Read the model definition and answer for the solid it produces. Units are mm, in the model's axes. Coordinates: 2 decimals unless noted, no trailing zeros. Answer as a JSON object with one key per item and string values. Group by question number.
1) Given pin 1 (6 mm diameter, centred on x = 0, y = 196, fed in from -Z), flat-ended and moving along its own axis, determine where the tip first touches the part or whether it passes through.
2) Consider L1, parallel to Y at x = 12, z = 1.55; L2, parallel to X at y = -224, z = 3; L3, parallel to X at y = -216, z = 3. Determine where each line is inside the solid, lowest interval first.
3) Section A-A on z = 4.2 is taken. Count the separate pieces of the cut face and the enclosed holes in it, and give its area (3 significant figures).
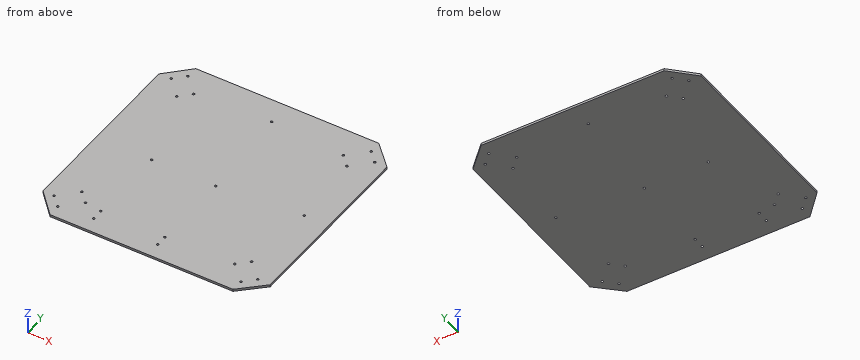
from build123d import *

# Parameters (mm, degrees)
SKETCH2_W           = 500
SKETCH2_H           = 500
BOSS_EXTRUDE1_DEPTH = 5
CUT_EXTRUDE1_DEPTH  = 5
SKETCH4_R           = 2.5
CUT_EXTRUDE4_DEPTH  = 6
SKETCH6_R           = 2.5
CUT_EXTRUDE5_DEPTH  = 6
SKETCH6_3_R         = 2.5
CUT_EXTRUDE6_DEPTH  = 6
SKETCH7_R           = 2.5
CUT_EXTRUDE7_DEPTH  = 6


with BuildPart() as part:
    # Sketch2 → Boss-Extrude1 (new body)
    with BuildSketch(Plane.XY):
        Rectangle(SKETCH2_W, SKETCH2_H)
    extrude(amount=BOSS_EXTRUDE1_DEPTH)

    # Sketch3 → Cut-Extrude1 (cut)
    with BuildSketch(Plane.XY.offset(5)):
        Polygon((-250, 250), (-250, 200.502525317), (-200.502525317, 250), align=None)
        Polygon((250, 250), (200.502525317, 250), (250, 200.502525317), align=None)
        Polygon((250, -202.085866883), (198.968285864, -250), (250, -250), align=None)
        Polygon((-202.085866883, -250), (-250, -198.968285864), (-250, -250), align=None)
    extrude(amount=-CUT_EXTRUDE1_DEPTH, mode=Mode.SUBTRACT)

    # Sketch4 → Cut-Extrude4 (cut, through all)
    with BuildSketch(Plane.XY.offset(5)):
        with Locations((-223.784016088, 201.333375785)):
            Circle(SKETCH4_R)
        with Locations((-201.333375785, 223.784016088)):
            Circle(SKETCH4_R)
        with Locations((-187.311960925, 163.528745219)):
            Circle(SKETCH4_R)
        with Locations((201.196010764, 222.516316525)):
            Circle(SKETCH4_R)
        with Locations((223.504797991, 199.924713826)):
            Circle(SKETCH4_R)
        with Locations((163.81847093, 185.606691548)):
            Circle(SKETCH4_R)
        with Locations((199.804611485, -223.79101951)):
            Circle(SKETCH4_R)
        with Locations((222.253825998, -201.338953508)):
            Circle(SKETCH4_R)
        with Locations((-187.65988085, -163.046698367)):
            Circle(SKETCH4_R)
        with Locations((-165.349658973, -185.636884284)):
            Circle(SKETCH4_R)
        with Locations((-225.035076637, -199.958696957)):
            Circle(SKETCH4_R)
        with Locations((-202.724854759, -222.548882874)):
            Circle(SKETCH4_R)
        with Locations((-164.861320622, 185.979385522)):
            Circle(SKETCH4_R)
        with Locations((186.127258156, 163.01508885)):
            Circle(SKETCH4_R)
        with Locations((185.10714798, -164.196993245)):
            Circle(SKETCH4_R)
        with Locations((162.657933466, -186.649059247)):
            Circle(SKETCH4_R)
    extrude(amount=-CUT_EXTRUDE4_DEPTH, mode=Mode.SUBTRACT)

    # Sketch6 → Cut-Extrude5 (cut, through all)
    with BuildSketch(Plane.XY.offset(5)):
        with Locations((-128, -216)):
            Circle(SKETCH6_R)
        with Locations((-128.2846398, -191)):
            Circle(SKETCH6_R)
        with Locations((-128.2846398, -16)):
            Circle(SKETCH6_R)
    extrude(amount=-CUT_EXTRUDE5_DEPTH, mode=Mode.SUBTRACT)

    # Sketch6<3> → Cut-Extrude6 (cut, through all)
    with BuildSketch(Plane.XY.offset(5)):
        with Locations((12, -215.71527189)):
            Circle(SKETCH6_3_R)
        with Locations((12, -191)):
            Circle(SKETCH6_3_R)
        with Locations((12, -16)):
            Circle(SKETCH6_3_R)
    extrude(amount=-CUT_EXTRUDE6_DEPTH, mode=Mode.SUBTRACT)

    # Sketch7 → Cut-Extrude7 (cut, through all)
    with BuildSketch(Plane.XY.offset(5)):
        with Locations((0, 196)):
            Circle(SKETCH7_R)
        with Locations((196, 0)):
            Circle(SKETCH7_R)
    extrude(amount=-CUT_EXTRUDE7_DEPTH, mode=Mode.SUBTRACT)


solid = part.part
Worked answers:
{
 "1": {"pin 1": "stops at z = 0"},
 "2": {"L1": "y = -250 to -218.22, -213.22 to -193.5, -188.5 to -18.5, -13.5 to 250", "L2": "x = -226.5 to -204.76, -200.69 to 197.31, 202.3 to 226.66", "L3": "x = -234.01 to -130.5, -125.5 to 9.52, 14.48 to 235.18"},
 "3": {"separate pieces": "1", "enclosed holes": "24", "area": "245,000 mm²"}
}
